from build123d import *

# Parameters (mm, degrees)
SKETCH053_R      = 1.6
SKETCH053_R_2    = 2
EXTRUDE045_DEPTH = 30
EXTRUDE044_DEPTH = 11


with BuildPart() as extrude045:
    # Sketch053 → Extrude045 (new body)
    with BuildSketch(Plane.XY.offset(23)):
        with Locations((-5, 2.5)):
            Circle(SKETCH053_R)
        with Locations((5, 2.5)):
            Circle(SKETCH053_R)
        with Locations((-5, -45.5)):
            Circle(SKETCH053_R)
        with Locations((5, -45.5)):
            Circle(SKETCH053_R)
        with Locations((0, -11.5)):
            Circle(SKETCH053_R_2)
    extrude(amount=-EXTRUDE045_DEPTH)


with BuildPart() as dummy_servo:
    # Sketch052 → Extrude044 (new body, symmetric)
    with BuildSketch(Plane(origin=(0, 0, 0), x_dir=(0, -1, 0), z_dir=(-1, 0, 0))):
        Polygon((-9, 2), (-9, 4), (2.5, 4), (2.5, 21.5), (20.5, 21.5), (20.5, 4), (52, 4), (52, 2), (19, 2), (19, 20), (4, 20), (4, 2), align=None)
    extrude(amount=EXTRUDE044_DEPTH, both=True)

    # Cut012: cut Extrude045
    add(extrude045.part, mode=Mode.SUBTRACT)


solid = dummy_servo.part
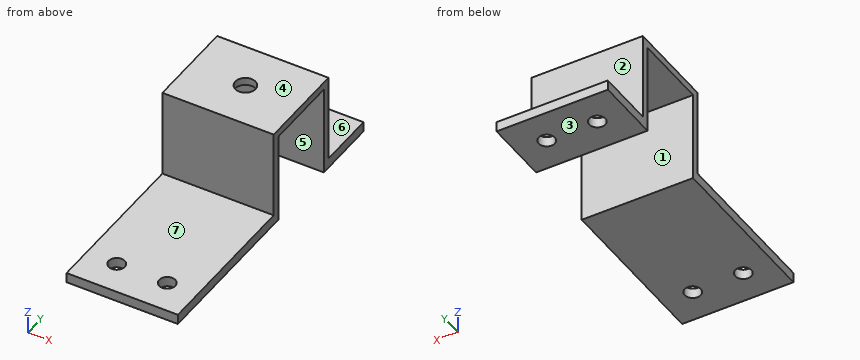
Could you check a few things on this model? Use its own coordinates, in mm. Face numbers are marked on the shaded views. A direction names the side the tool comes from. Give positions to 0.01 mm unless a question says otherwise; leave off trailing zeros. Loops run counter-clockwise (first coordinate to the right, second up) from the corner with the lowest first, then second, coordinate; pieces in that order, holes last. Notation, with made-up numbers: M 38,-19 L 88,-19 A10 cw 88,-10 Z; hole C 69.25,38.25 d9. An arc over 180 degrees is marked long. Answer as a JSON object with one key per item and string values.
Q1. For P1, Ø3, axis at x = 4, y = 1, coming from the +Z side; P2, Ø2, axis at x = -2.5, z = 13, coming from the +Y side, each with a flat end and sliding along its axis, tell me the tip position at first contact or that it passes through.
Values found:
{"P1": "stops at z = 4", "P2": "stops at y = -2.5"}
Q2. If I drill on probe 1 along Y at (x, z) = (5, 2.8); probe 2 along Y at (x, z) = (-5, 14.5); probe 3 along Z at (x, y) = (8, 3.5), over which ranges is the centre line in solid material (lowest first)? Write a range as [from, to].
Values found:
{"probe 1": "y = [-52, -47.1], [-43.9, -19], [-4, 0.9], [4.1, 9]", "probe 2": "y = [-20.5, -19], [-4, -2.5]", "probe 3": "z = [2, 4]"}
Q3. Suppose I cut it at C-C, the plane x = 5. List the corners of the cut face in (y, z) for me, plus the area to 3 significant figures.
Values found:
{"outline": "M -52,2 L -47.1,2 L -47.1,4 L -52,4 Z; M -43.9,2 L -19,2 L -19,20 L -4,20 L -4,2 L 0.9,2 L 0.9,4 L -2.5,4 L -2.5,21.5 L -20.5,21.5 L -20.5,4 L -43.9,4 Z; M 4.1,2 L 9,2 L 9,4 L 4.1,4 Z", "area": "154 mm²"}
Q4. Suppose I cut it at B-B, the plane z = 10.25. List the corners of the cut face in (x, y) for me, plus the area to 3 significant figures.
Values found:
{"outline": "M -11,-20.5 L 11,-20.5 L 11,-19 L -11,-19 Z; M -11,-4 L 11,-4 L 11,-2.5 L -11,-2.5 Z", "area": "66.0 mm²"}
Q5. If we mould it in two halves opening along Y, with no side actions, what happens to the marked faces 1, 2 and 3? For each: pulls with the +Y half, pulls with the -Y half, needs draft (parallel to the pull), parting line crosses it, or undercut.
Values found:
{"face 1": "undercut", "face 2": "pulls with the +Y half", "face 3": "needs draft"}
Q6. Suppose I cut it at A-A, the plane y = 2.5. List the corners of the cut face in (x, z) for me, plus the area to 3 significant figures.
Values found:
{"outline": "M -11,2 L -6.6,2 L -6.6,4 L -11,4 Z; M -3.4,2 L 3.4,2 L 3.4,4 L -3.4,4 Z; M 6.6,2 L 11,2 L 11,4 L 6.6,4 Z", "area": "31.2 mm²"}
Q7. For the marked faces 4, 5, 6 and 7, which set-ups out of +Z, -Z, +X, -X, +Y, -Y let a thin tool reach every point of the face, with its end or its side?
Values found:
{"face 4": "+Z, +X, -X, +Y, -Y", "face 5": "-Z, +X, -X", "face 6": "+Z, +X, -X, +Y", "face 7": "+Z, +X, -X, -Y"}
Q8. Suppose I cut it at D-D, the plane y = -11.5. List the corners of the cut face in (x, z) for me, plus the area to 3 significant figures.
Values found:
{"outline": "M -11,20 L -2,20 L -2,21.5 L -11,21.5 Z; M 2,20 L 11,20 L 11,21.5 L 2,21.5 Z", "area": "27.0 mm²"}
